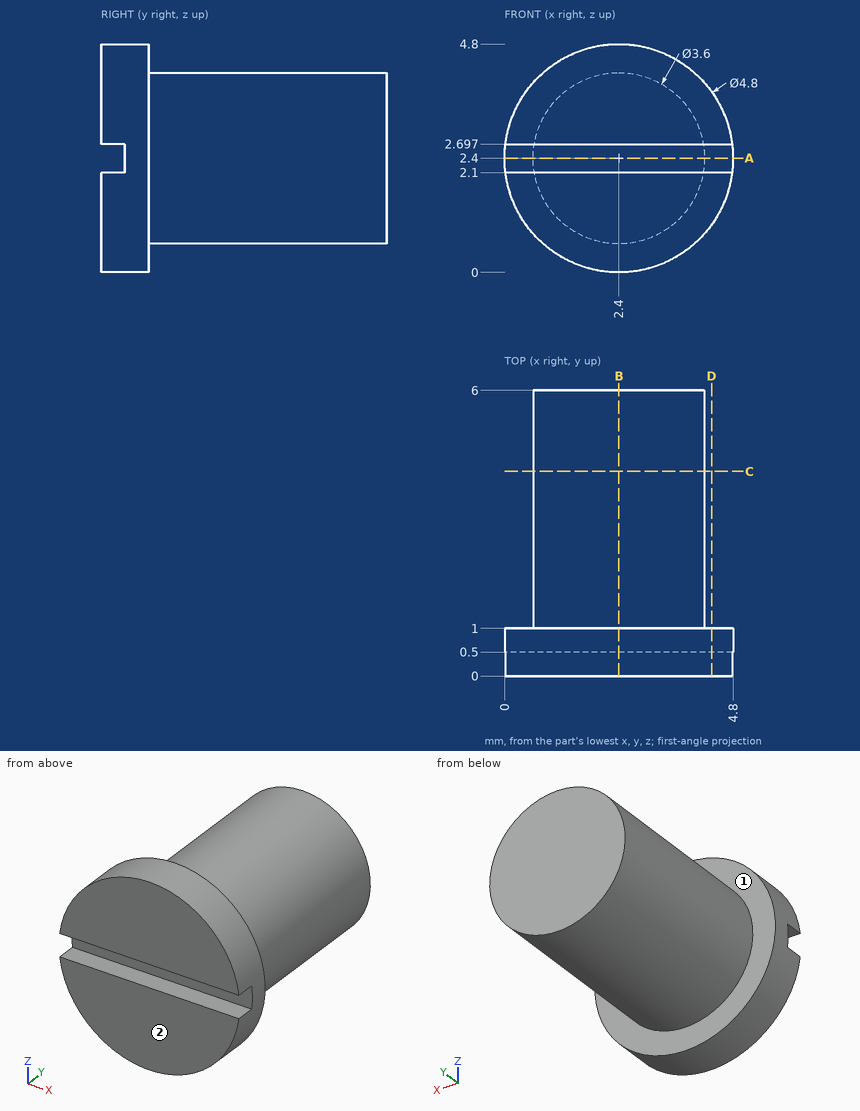
The drawing under review shows one solid part. Ordinate dimensions are in mm from its lowest x, y, z. A direction names the side the tool comes from. Round coordinates to 2 decimals unless told otherwise and drop trailing zeros. Loops run counter-clockwise (first coordinate to the right, second up) from the corner with the lowest first, then second, coordinate; pieces in that order, holes last.
Item 1: Take a section at A-A (z = 2.4). Write out the cut boundary in (x, y).
Determined:
outline: (0, 0.5) - (4.8, 0.5) - (4.8, 1) - (4.2, 1) - (4.2, 6) - (0.6, 6) - (0.6, 1) - (0, 1) - close
Item 2: For the marked faces 1 and 2, list the 3-axis set-ups (+Z, -Z, +X, -X, +Y, -Y) from which the entire face can be reached by the end or side of a thin tool; tool diameter is ignored.
Determined:
face 1: +Y
face 2: +Z, -Z, +X, -X, -Y
Item 3: Take a section at B-B (x = 2.4). Write out the cut boundary in (y, z), then the cut area to 3 significant figures.
Determined:
outline: (0, 0) - (1, 0) - (1, 0.6) - (6, 0.6) - (6, 4.2) - (1, 4.2) - (1, 4.8) - (0, 4.8) - (0, 2.7) - (0.5, 2.7) - (0.5, 2.1) - (0, 2.1) - close
area: 22.5 mm2
Item 4: Take a section at C-C (y = 4.3). Write out the cut boundary in (x, z).
Determined:
outline: circle Ø3.6 at (2.4, 2.4)
Item 5: For line 1 (Z direction, x = 3.4, y = 0.35); line 2 (Z direction, x = 2.35, y = 2.6); line 3 (X direction, y = 0.65, z = 2.3), list the stretches that pass through material, from the lowest coordinate up.
Determined:
line 1: z = 0.22 to 2.1, 2.7 to 4.58
line 2: z = 0.6 to 4.2
line 3: x = 0 to 4.8
Item 6: Take a section at D-D (x = 4.35). Write out the cut boundary in (y, z), then the cut area to 3 significant figures.
Determined:
outline: (0, 1) - (1, 1) - (1, 3.8) - (0, 3.8) - (0, 2.7) - (0.5, 2.7) - (0.5, 2.1) - (0, 2.1) - close
area: 2.50 mm2
Item 7: Clearance check with flat-ended pins moving along their axes: pin 1 Ø0.6 at (x, y) = (1.5, 0) entering from -Z; pin 2 Ø0.6 at (x, y) = (2, 0) entering from +Z. State where each tip first meets the part, or that it passes through.
Determined:
pin 1: stops at z = 0.08
pin 2: stops at z = 4.8
